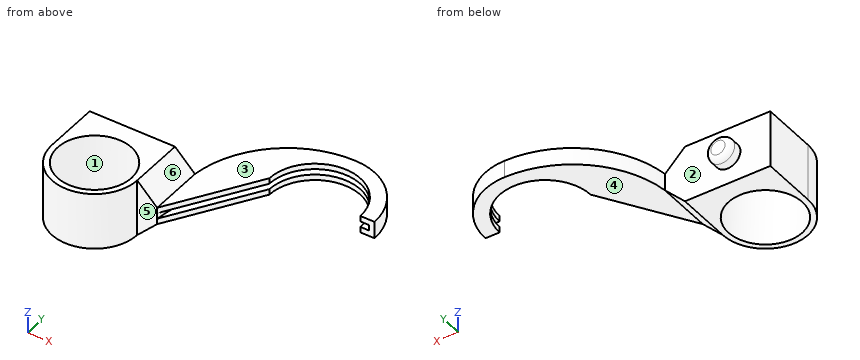
```python
from build123d import *

# Parameters (mm, degrees)
SKETCH1_R           = 13
BOSS_EXTRUDE1_DEPTH = 10
BOSS_EXTRUDE2_DEPTH = 19.5
BOSS_EXTRUDE3_DEPTH = 3
BOSS_EXTRUDE4_DEPTH = 2
SKETCH5_R           = 4.5
BOSS_EXTRUDE5_DEPTH = 5
FILLET1_R           = 2


with BuildPart() as part:
    # Sketch1 → Boss-Extrude1 (new, symmetric)
    with BuildSketch(Plane.XY):
        with BuildLine():
            Line((-15, 0), (-15, 19.5))
            Line((-15, 19.5), (15, 19.5))
            Line((15, 19.5), (15, 0))
            ThreePointArc((15, 0), (0, -15), (-15, 0))
        make_face()
        Circle(SKETCH1_R, mode=Mode.SUBTRACT)
    extrude(amount=BOSS_EXTRUDE1_DEPTH, both=True)

    # Sketch3 → Boss-Extrude2 (add)
    with BuildSketch(Plane(origin=(0, 19.5, 0), x_dir=(1, 0, 0), z_dir=(0, 1, 0))):
        Polygon((15, 10), (22, 3), (22, -3), (15, -10), align=None)
    extrude(amount=-BOSS_EXTRUDE2_DEPTH)

    # Sketch2 → Boss-Extrude3 (add, symmetric)
    with BuildSketch(Plane.XY):
        with BuildLine():
            Line((78, 30), (76, 30))
            ThreePointArc((76, 30), (64.47643512, 47.467195479), (43.88390338, 43.74656355))
            ThreePointArc((43.88390338, 43.74656355), (29.130686528, 23.779839726), (22, 0))
            Line((22, 0), (22, 19.5))
            ThreePointArc((22, 19.5), (33.456157918, 41.965380092), (57, 51))
            ThreePointArc((57, 51), (71.849242405, 44.849242405), (78, 30))
        make_face()
    extrude(amount=BOSS_EXTRUDE3_DEPTH, both=True)


with BuildPart() as body_2:
    # Sketch4 → Boss-Extrude4 (new body)
    with BuildSketch(Plane.XY.offset(3)):
        with BuildLine():
            Line((73, 30), (76, 30))
            ThreePointArc((76, 30), (64.47643512, 47.467195479), (43.88390338, 43.74656355))
            ThreePointArc((43.88390338, 43.74656355), (29.130686528, 23.779839726), (22, 0))
            Line((22, 0), (41, 30))
            ThreePointArc((41, 30), (57, 46), (73, 30))
        make_face()
    extrude(amount=-BOSS_EXTRUDE4_DEPTH)


with BuildPart() as body_3:
    # Mirror1: mirrored copy
    add(body_2.part.mirror(Plane.XY))


with BuildPart() as body_2_1:
    add(body_2.part)

    # Combine2: union body 3, part
    add(body_3.part)
    add(part.part)

    # Sketch5 → Boss-Extrude5 (add, symmetric)
    with BuildSketch(Plane(origin=(0, 19.5, 0), x_dir=(1, 0, 0), z_dir=(0, 1, 0))):
        with Locations(Location((0, 0, 0), (0, 0, 90))):
            Circle(SKETCH5_R)
    extrude(amount=BOSS_EXTRUDE5_DEPTH, both=True)

    # Fillet1
    fillet1_edges = [body_2_1.edges().sort_by_distance(p)[0] for p in [
        (0, 24.5, 4.5),
    ]]
    fillet(fillet1_edges, radius=FILLET1_R)


solid = body_2_1.part
```
Work out the finished part from the listing and answer in its coordinate system (mm). Face numbers are marked on the shaded views. A direction names the side the tool comes from. Round coordinates to 2 decimals unless told otherwise and drop trailing zeros. Order: outer loops, then holes, each group sorted by start corner. A loop starts at its lowest first (then second) coordinate and runs counter-clockwise, first axis right, second up.
Q1. Given pin 1 Ø1 at (x, y) = (25, 6.5) entering from -Z; pin 2 Ø5.5 at (x, z) = (76.5, 0) entering from -Y; pin 3 Ø5.5 at (x, z) = (20, -4) entering from -Y; pin 4 Ø21 at (x, y) = (0, 0) entering from +Z, each flat-ended and moving along its own axis, determine where each tip first touches the part or whether it passes through.
Solution:
pin 1: stops at z = -3
pin 2: stops at y = 30
pin 3: stops at y = 0
pin 4: passes through
Q2. A cutting plane is placed at D-D, the plane x = 18.5. Determine the outline of the cut face in (y, z), then the cut area to 4 significant figures.
Solution:
outline: (0, -6.5) - (19.5, -6.5) - (19.5, 6.5) - (0, 6.5) - close
area: 253.5 mm2
Q3. A cutting plane is placed at A-A, the plane x = 0. Determine the outline of the cut face in (y, z).
Solution:
outline: (-15, -10) - (-13, -10) - (-13, 10) - (-15, 10) - close; (13, -10) - (19.5, -10) - (19.5, -4.5) - (22.5, -4.5) arc R2 ccw to (24.5, -2.5) - (24.5, 2.5) arc R2 ccw to (22.5, 4.5) - (19.5, 4.5) - (19.5, 10) - (13, 10) - close
Q4. Find the intervals of material crossed by line 1 along Y through (x, z) = (0, 5.75); line 2 along Y through (x, z) = (0, 2.25); line 3 along Y through (x, z) = (20, -1), in increasing order.
Solution:
line 1: y = -15 to -13, 13 to 19.5
line 2: y = -15 to -13, 13 to 24.5
line 3: y = 0 to 19.5
Q5. A cutting plane is placed at B-B, the plane y = 3. Determine the outline of the cut face in (x, z), then the cut area to 3 significant figures.
Solution:
outline: (-15, -10) - (-12.65, -10) - (-12.65, 10) - (-15, 10) - close; (12.65, -10) - (15, -10) - (22, -3) - (23.9, -3) - (23.9, -1) - (22.42, -1) - (22.42, 1) - (23.9, 1) - (23.9, 3) - (22, 3) - (15, 10) - (12.65, 10) - close
area: 193 mm2
Q6. A tool of negligible diameter and unlimited length cuts with its end or side. For the marked faces 4, 5 and 6, from which of +Z, -Z, +X, -X, +Y, -Y can it reach the whole face along a straight path? Write none if from no direction.
Solution:
face 4: -Z, +X, +Y, -Y
face 5: +Z, -Z, +X, -Y
face 6: +Z, +X, +Y, -Y
Q7. A cutting plane is placed at C-C, the plane z = 0. Determine the outline of the cut face in (x, y).
Solution:
outline: (-15, 0) arc R15 ccw to (15, 0) - (22, 0) arc R72.31 cw to (43.88, 43.75) arc R19 cw to (76, 30) - (78, 30) arc R21 ccw to (57, 51) arc R35.19 ccw to (22, 19.5) - (4.5, 19.5) - (4.5, 22.5) arc R2 ccw to (2.5, 24.5) - (-2.5, 24.5) arc R2 ccw to (-4.5, 22.5) - (-4.5, 19.5) - (-15, 19.5) - close; hole circle Ø26 at (0, 0)
Q8. The mould has two halves that part along Y. Classify the marked faces 1, 2 and 3: pulls with the +Y half, pulls with the -Y half, needs draft (parallel to the pull), parting line crosses it, or undercut.
Solution:
face 1: undercut
face 2: pulls with the +Y half
face 3: needs draft
